from build123d import *

# Parameters (mm, degrees)
F0_W     = 7
F0_H     = 5
F1_DEPTH = 3
F2_R     = 1.99999


# Not quite as in the source:
# - a fillet or chamfer is up to 0.001 mm smaller than in the source, because OpenCascade refuses the exact size
# - a feature names something its author has since deleted; it is built from what else it names


with BuildPart() as f1:
    # F0 (on Top) → F1 (new body)
    with BuildSketch(Plane.XY):
        Polygon((25, 0), (0, 0), (-12, 37), (-16, 37), (-16, -4), (29, -4), (29, 11), (25, 11), align=None)
        with Locations((-9.5, 1.5)):
            Rectangle(F0_W, F0_H, mode=Mode.SUBTRACT)
        Polygon((-13, 8.7756748306), (-13, 30.3590081639), (-6, 8.7756748306), align=None, mode=Mode.SUBTRACT)
    extrude(amount=F1_DEPTH)

    # F2 (radius 2 in the source; OpenCascade refuses exactly that, so slightly less here)
    f2_edges = [f1.edges().sort_by_distance(p)[0] for p in [
        (-16, -4, 1.5),
        (25, 0, 1.5),
        (-12, 37, 1.5),
        (29, 11, 1.5),
        (0, 0, 1.5),
        (-16, 37, 1.5),
        (29, -4, 1.5),
        (25, 11, 1.5),
    ]]
    fillet(f2_edges, radius=F2_R)


solid = f1.part
Could you check a few things on this model? Use its own coordinates, in mm. A direction names the side the tool comes from. Give positions to 0.01 mm unless a question says otherwise; leave off trailing zeros. Order: outer loops, then holes, each group sorted by start corner. A loop starts at its lowest first (then second) coordinate and runs counter-clockwise, first axis right, second up.
1. We'd pull the mould along X, two halves only. Please class faces 1 (the cylindrical face through (28.43, -3.4, 1.52)), 2 (the flat face through (-9, 8.776, 1)), 3 (the flat face through (-9.55, 19.72, 1.48)), 4 (the flat face through (-4, 11, 0)): pulls with the +X half, pulls with the -X half, needs draft (parallel to the pull), parting line crosses it, or undercut.
2. Suppose I cut it at C-C (y = 4.5). List the corners of the cut face in (x, z) for me, plus the area to 3 significant figures.
3. Suppose I cut it at D-D (x = 22.5). List the corners of the cut face in (y, z) for me.
4. Suppose I cut it at B-B (y = 10). List the corners of the cut face in (x, z) for me.
5. Will these pins go through, and if not, where does the flat tip stop? P1, Ø0.9, axis at x = 12, z = 2, coming from the +Y side; P2, Ø1, axis at x = -9, y = 15.5, coming from the -Z side; P3, Ø10, axis at x = -8, y = 7.5, coming from the -Z side.
6. I need wall thicknesses on L1, parallel to X at y = -0.5, z = 2.6; L2, parallel to X at y = 2, z = 2.45; L3, parallel to X at y = 9, z = 1.35. Which ranges of each line are inside material? Lowest first, please.
7. Suppose I cut it at A-A (z = 1.8). Give the number of separate pieces and of enclosed holes in the cut face, plus the area to 3 significant figures.
8. For faces 5 (the cylindrical face through (24.4, 0.57, 1.52)), 6 (the flat face through (29, 3, 1)), 7 (the flat face through (-10, 4, 1)), which set-ups out of +Z, -Z, +X, -X, +Y, -Y let a thin tool reach every point of the face, with its end or its side?
Solved:
1. face 1: pulls with the +X half
1. face 2: undercut
1. face 3: undercut
1. face 4: needs draft
2. outline: (-16, 0) - (-1.46, 0) - (-1.46, 3) - (-16, 3) - close; (25, 0) - (29, 0) - (29, 3) - (25, 3) - close
2. area: 55.6 mm2
3. outline: (-4, 0) - (0, 0) - (0, 3) - (-4, 3) - close
4. outline: (-16, 0) - (-13, 0) - (-13, 3) - (-16, 3) - close; (-6.4, 0) - (-3.24, 0) - (-3.24, 3) - (-6.4, 3) - close; (25.27, 0) - (28.73, 0) - (28.73, 3) - (25.27, 3) - close
5. P1: stops at y = 0
5. P2: passes through
5. P3: stops at z = 0
6. L1: x = -16 to -13, -6 to 29
6. L2: x = -16 to -13, -6 to -0.65, 25 to 29
6. L3: x = -16 to -13, -6.07 to -2.92, 25 to 29
7. separate pieces: 1
7. enclosed holes: 2
7. area: 480 mm2
8. face 5: +Z, -Z, +Y
8. face 6: +Z, -Z, +X, +Y, -Y
8. face 7: +Z, -Z
